```python
from build123d import *

# Parameters (mm, degrees)
SKETCH_1_W          = 180
SKETCH_1_H          = 140
SKETCH_1_W_2        = 71
SKETCH_1_H_2        = 70
SKETCH_1_W_3        = 10
SKETCH_1_H_3        = 9.5
EXTRUDE_1_DEPTH     = 1.5
FILLET_1_R          = 20
FILLET_2_R          = 5
SKETCH_2_W          = 12.5
SKETCH_2_H          = 40
CUT_EXTRUDE_1_DEPTH = 3
SKETCH_3_W          = 3
SKETCH_3_H          = 10
EXTRUDE_2_DEPTH     = 3
CUT_EXTRUDE_2_DEPTH = 3
SKETCH_6_R          = 2.25
SKETCH_6_R_2        = 1.25
SKETCH_6_R_3        = 2
CUT_EXTRUDE_3_DEPTH = 10


with BuildPart() as part:
    # 草图1 → 凸台-拉伸1 (new, symmetric)
    # profile 1 of 5: a face of its own
    with BuildSketch(Plane.XY):
        Rectangle(SKETCH_1_W, SKETCH_1_H)
        with Locations((2, 0)):
            Rectangle(SKETCH_1_W_2, SKETCH_1_H_2, mode=Mode.SUBTRACT)
    # profile 2 of 5: a face of its own
    with BuildSketch(Plane.XY):
        with Locations((-28.5, -30.25)):
            Rectangle(SKETCH_1_W_3, SKETCH_1_H_3)
    # profile 3 of 5: a face of its own
    with BuildSketch(Plane.XY):
        with Locations((32.5, -30.25)):
            Rectangle(SKETCH_1_W_3, SKETCH_1_H_3)
    # profile 4 of 5: a face of its own
    with BuildSketch(Plane.XY):
        with Locations((32.5, 30.25)):
            Rectangle(SKETCH_1_W_3, SKETCH_1_H_3)
    # profile 5 of 5: a face of its own
    with BuildSketch(Plane.XY):
        with Locations((-28.5, 30.25)):
            Rectangle(SKETCH_1_W_3, SKETCH_1_H_3)
    extrude(amount=EXTRUDE_1_DEPTH, both=True)

    # 圆角1
    fillet_1_edges = [part.edges().sort_by_distance(p)[0] for p in [
        (90, -70, 0),
        (-90, -70, 0),
        (-90, 70, 0),
        (90, 70, 0),
    ]]
    fillet(fillet_1_edges, radius=FILLET_1_R)

    # 圆角2
    fillet_2_edges = [part.edges().sort_by_distance(p)[0] for p in [
        (-23.5, 25.5, 0),
        (-23.5, -25.5, 0),
        (27.5, -25.5, 0),
        (27.5, 25.5, 0),
    ]]
    fillet(fillet_2_edges, radius=FILLET_2_R)

    # 草图2 → 切除-拉伸1 (cut)
    with BuildSketch(Plane.XY.offset(1.5)):
        with Locations((58.75, 0)):
            Rectangle(SKETCH_2_W, SKETCH_2_H)
    cut_extrude_1 = extrude(amount=-CUT_EXTRUDE_1_DEPTH, mode=Mode.SUBTRACT)

    # 草图3 → 凸台-拉伸2 (add)
    with BuildSketch(Plane.XY.offset(1.5)):
        with Locations((-32, 12.5)):
            Rectangle(SKETCH_3_W, SKETCH_3_H)
        with Locations((36, -12.5)):
            Rectangle(SKETCH_3_W, SKETCH_3_H)
        with Locations((-32, -12.5)):
            Rectangle(SKETCH_3_W, SKETCH_3_H)
        with Locations((36, 12.5)):
            Rectangle(SKETCH_3_W, SKETCH_3_H)
    extrude(amount=-EXTRUDE_2_DEPTH)

    # 草图5 → 切除-拉伸2 (cut)
    with BuildSketch(Plane.XY.offset(1.5)):
        Polygon((-30.5, 14.75), (-36.5, 14.75), (-36.5, 16.75), (-41.5, 16.75), (-41.5, 14.75), (-45.5, 14.75), (-45.5, 10.25), (-41.5, 10.25), (-41.5, 8.25), (-36.5, 8.25), (-36.5, 10.25), (-30.5, 10.25), align=None)
        Polygon((-36.5, -10.25), (-30.5, -10.25), (-30.5, -14.75), (-36.5, -14.75), (-36.5, -16.75), (-41.5, -16.75), (-41.5, -14.75), (-45.5, -14.75), (-45.5, -10.25), (-41.5, -10.25), (-41.5, -8.25), (-36.5, -8.25), align=None)
        Polygon((40.5, -8.25), (40.5, -10.25), (34.5, -10.25), (34.5, -14.75), (40.5, -14.75), (40.5, -16.75), (45.5, -16.75), (45.5, -14.75), (49.5, -14.75), (49.5, -10.25), (45.5, -10.25), (45.5, -8.25), align=None)
        Polygon((40.5, 10.25), (34.5, 10.25), (34.5, 14.75), (40.5, 14.75), (40.5, 16.75), (45.5, 16.75), (45.5, 14.75), (49.5, 14.75), (49.5, 10.25), (45.5, 10.25), (45.5, 8.25), (40.5, 8.25), align=None)
    extrude(amount=-CUT_EXTRUDE_2_DEPTH, mode=Mode.SUBTRACT)

    # 草图6 → 切除-拉伸3 (cut)
    with BuildSketch(Plane.XY.offset(1.5)):
        with Locations((-80, 50)):
            Circle(SKETCH_6_R)
        with Locations((80, 50)):
            Circle(SKETCH_6_R)
        with Locations((80, -50)):
            Circle(SKETCH_6_R)
        with Locations((-80, -50)):
            Circle(SKETCH_6_R)
        with Locations((-22.605, -41)):
            Circle(SKETCH_6_R_2)
        with Locations((22.605, -41)):
            Circle(SKETCH_6_R_2)
        with Locations((22.605, -59)):
            Circle(SKETCH_6_R_2)
        with Locations((-22.605, -59)):
            Circle(SKETCH_6_R_2)
        with Locations((22.605, 59)):
            Circle(SKETCH_6_R_2)
        with Locations((22.605, 41)):
            Circle(SKETCH_6_R_2)
        with Locations((-22.605, 41)):
            Circle(SKETCH_6_R_2)
        with Locations((-22.605, 59)):
            Circle(SKETCH_6_R_2)
        with Locations((0, 50)):
            Circle(SKETCH_6_R_3)
        with Locations((40, 50)):
            Circle(SKETCH_6_R_3)
        with Locations((-40, 50)):
            Circle(SKETCH_6_R_3)
        with Locations((0, -50)):
            Circle(SKETCH_6_R_3)
        with Locations((40, -50)):
            Circle(SKETCH_6_R_3)
        with Locations((-40, -50)):
            Circle(SKETCH_6_R_3)
        with Locations((-80, 0)):
            Circle(SKETCH_6_R)
        with Locations((80, 0)):
            Circle(SKETCH_6_R)
    extrude(amount=-CUT_EXTRUDE_3_DEPTH, mode=Mode.SUBTRACT)

    # 镜向1: 切除-拉伸1 across plane
    add(cut_extrude_1.mirror(Plane(origin=(0, 0, 0), x_dir=(0, 0, 1), z_dir=(1, 0, 0))), mode=Mode.SUBTRACT)


solid = part.part
```
The model under review builds one solid part; all positions refer to its coordinate system, in mm. A direction names the side the tool comes from. Round coordinates to 2 decimals unless told otherwise and drop trailing zeros. Order: outer loops, then holes, each group sorted by start corner. A loop starts at its lowest first (then second) coordinate and runs counter-clockwise, first axis right, second up.
(1) Mouldability with a two-part tool opening along X and no side actions: class faces 1 (the face through (39, 1, 1.5)), 2 (the face through (-83.986, 64.297, -0.021)), 3 (the face through (-25, 26.93, 0.02)) as released by +X, released by -X, zero draft, split by the parting line, or undercut.
Working result:
face 1: zero draft
face 2: released by -X
face 3: undercut
(2) Take a section at A-A, the plane x = -8. State the section outline as (y, z) points.
Working result:
outline: (-70, -1.5) - (-35, -1.5) - (-35, 1.5) - (-70, 1.5) - close; (35, -1.5) - (70, -1.5) - (70, 1.5) - (35, 1.5) - close
(3) Take a section at C-C, the plane x = -80. State the section outline as (y, z) points, plus the area to 3 significant figures.
Working result:
outline: (-67.32, -1.5) - (-52.25, -1.5) - (-52.25, 1.5) - (-67.32, 1.5) - close; (-47.75, -1.5) - (-2.25, -1.5) - (-2.25, 1.5) - (-47.75, 1.5) - close; (2.25, -1.5) - (47.75, -1.5) - (47.75, 1.5) - (2.25, 1.5) - close; (52.25, -1.5) - (67.32, -1.5) - (67.32, 1.5) - (52.25, 1.5) - close
area: 363 mm2
(4) Wall thickness on L1, parallel to Y at x = 35, z = -1.2; L2, parallel to Y at x = 40, z = -0.35; L3, parallel to X at y = -6.5, z = 0.35: over which ranges is each line inside the solid? List them lowest first.
Working result:
L1: y = -70 to -25.5, -17.5 to -14.75, -10.25 to -7.5, 7.5 to 10.25, 14.75 to 17.5, 25.5 to 70
L2: y = -70 to -52, -48 to -14.75, -10.25 to 10.25, 14.75 to 48, 52 to 70
L3: x = -90 to -65, -52.5 to -33.5, 37.5 to 52.5, 65 to 90
(5) Take a section at D-D, the plane z = -0.65. Count the separate pieces of the cut face and the enclosed holes in it, plus the area to 3 significant figures.
Working result:
separate pieces: 1
enclosed holes: 23
area: 18,800 mm2
(6) Tool access review of faces 4 (the face through (-24.93, -27, -0.02)), 5 (the face through (-83.986, -64.297, 0.021)): name each direction out of +Z, -Z, +X, -X, +Y, -Y from which nothing blocks a thin tool from reaching the whole face with its end or side.
Working result:
face 4: +Z, -Z
face 5: +Z, -Z, -X, -Y
(7) Take a section at B-B, the plane y = 0. State the section outline as (x, z) points.
Working result:
outline: (-90, -1.5) - (-82.25, -1.5) - (-82.25, 1.5) - (-90, 1.5) - close; (-77.75, -1.5) - (-65, -1.5) - (-65, 1.5) - (-77.75, 1.5) - close; (-52.5, -1.5) - (-33.5, -1.5) - (-33.5, 1.5) - (-52.5, 1.5) - close; (37.5, -1.5) - (52.5, -1.5) - (52.5, 1.5) - (37.5, 1.5) - close; (65, -1.5) - (77.75, -1.5) - (77.75, 1.5) - (65, 1.5) - close; (82.25, -1.5) - (90, -1.5) - (90, 1.5) - (82.25, 1.5) - close
